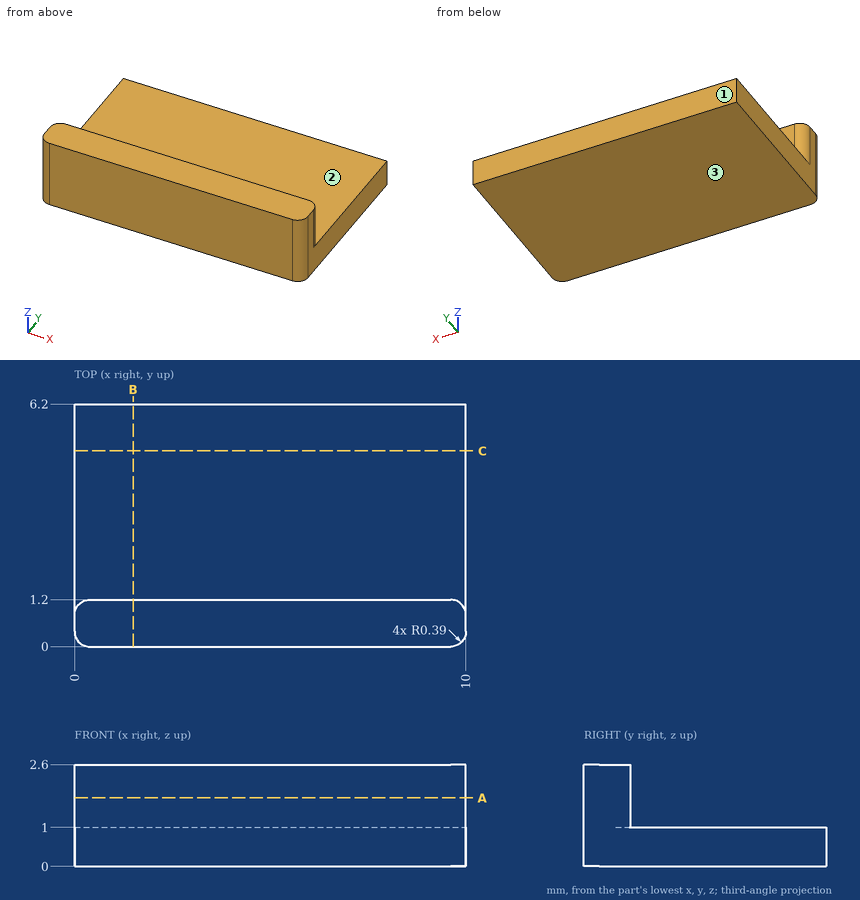
Source: three-view drawing plus pictorial views. Frame: mm from the lowest corner of the part. Give positions to 0.01 mm unless a question says otherwise; leave off trailing zeros. Loops run counter-clockwise (first coordinate to the right, second up) from the corner with the lowest first, then second, coordinate; pieces in that order, holes last. Notation, with made-up numbers: M -26,12.5 L 6,12.5 A28 ccw 6,42.5 Z; hole C -1,77 d4. An arc over 180 degrees is marked long. Put each result on its own line as item: value.
Q1. Section B-B (x = 1.5). Return the cut outline in (y, z).
Response values:
outline: M 0,0 L 6.2,0 L 6.2,1 L 1.2,1 L 1.2,2.6 L 0,2.6 Z
Q2. Line query: probe 1 along Z at (x, y) = (9.75, 4); probe 2 along Y at (x, z) = (9, 2.3); probe 3 along X at (y, z) = (1, 1.2). Output: solid intervals per line, ascending. Write a range as [from, to].
Response values:
probe 1: z = [0, 1]
probe 2: y = [0, 1.2]
probe 3: x = [0.05, 9.95]
Q3. Section A-A (z = 1.75). Return the cut outline in (x, y), and give its area (3 significant figures).
Response values:
outline: M 0,0.39 A0.39 ccw 0.39,0 L 9.61,0 A0.39 ccw 10,0.39 L 10,0.81 A0.39 ccw 9.61,1.2 L 0.39,1.2 A0.39 ccw 0,0.81 Z
area: 11.9 mm²
Q4. Section C-C (y = 5). Return the cut outline in (x, z).
Response values:
outline: M 0,0 L 10,0 L 10,1 L 0,1 Z
Q5. Mould query, pull axis Z, two halves, no side actions, for the marked faces 1, 2 and 3. Classes: released by +Z, released by -Z, zero draft, split by the parting line, or undercut.
Response values:
face 1: zero draft
face 2: released by +Z
face 3: released by -Z
